Could you check a few things on this model? Use its own coordinates, in mm. Face numbers are marked on the shaded views. A direction names the side the tool comes from. Round coordinates to 2 decimals unless told otherwise and drop trailing zeros. Loops run counter-clockwise (first coordinate to the right, second up) from the corner with the lowest first, then second, coordinate; pieces in that order, holes last. Notation, with made-up numbers: (-19.75, 75) -> (39.25, 75) arc R4 ccw to (39.25, 82) -> close; hole circle Ø3 at (11, 81). An arc over 180 degrees is marked (long way). One line per item, written item: value.
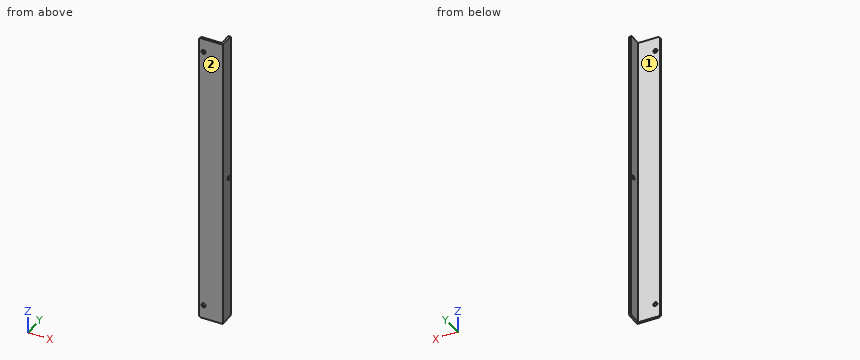
```python
from build123d import *

# Parameters (mm, degrees)
BOSS_EXTRUDE1_DEPTH = 750
CUT_EXTRUDE1_REACH  = 755.21
SKETCH4_R           = 5.25
CUT_EXTRUDE2_REACH  = 755.077
SKETCH5_R           = 5.25
CHAMFER1_SIZE       = 4


with BuildPart() as part:
    # Sketch1 → Boss-Extrude1 (new body)
    with BuildSketch(Plane.XY):
        Polygon((0, 0), (-60, 0), (-60, 5), (-5, 5), (-5, 40), (0, 40), align=None)
    extrude(amount=BOSS_EXTRUDE1_DEPTH)

    # Sketch4 → Cut-Extrude1 (cut, up to next)
    with BuildSketch(Plane(origin=(0, 5, 0), x_dir=(1, 0, 0), z_dir=(0, 1, 0)), mode=Mode.PRIVATE) as cut_extrude1_sk1:
        with Locations(Location((-48, -35, 0), (0, 0, 270))):
            Circle(SKETCH4_R)
    cut_extrude1_tool1 = extrude(cut_extrude1_sk1.sketch, amount=-CUT_EXTRUDE1_REACH, mode=Mode.PRIVATE) & part.part
    # Sketch4 → Cut-Extrude1 (cut, up to next)
    with BuildSketch(Plane(origin=(0, 5, 0), x_dir=(1, 0, 0), z_dir=(0, 1, 0)), mode=Mode.PRIVATE) as cut_extrude1_sk2:
        with Locations(Location((-48, -715, 0), (0, 0, 180))):
            Circle(SKETCH4_R)
    cut_extrude1_tool2 = extrude(cut_extrude1_sk2.sketch, amount=-CUT_EXTRUDE1_REACH, mode=Mode.PRIVATE) & part.part
    add(cut_extrude1_tool1.solids().sort_by_distance((-48, 5, 35))[0], mode=Mode.SUBTRACT)
    add(cut_extrude1_tool2.solids().sort_by_distance((-48, 5, 715))[0], mode=Mode.SUBTRACT)

    # Sketch5 → Cut-Extrude2 (cut, up to next)
    with BuildSketch(Plane.ZY.offset(5), mode=Mode.PRIVATE) as cut_extrude2_sk1:
        with Locations(Location((375, 28, 0), (0, 0, 270))):
            Circle(SKETCH5_R)
    cut_extrude2_tool1 = extrude(cut_extrude2_sk1.sketch, amount=-CUT_EXTRUDE2_REACH, mode=Mode.PRIVATE) & part.part
    add(cut_extrude2_tool1.solids().sort_by_distance((-5, 28, 375))[0], mode=Mode.SUBTRACT)

    # Chamfer1
    chamfer1_edges = [part.edges().sort_by_distance(p)[0] for p in [
        (-60, 2.5, 750),
        (-60, 2.5, 0),
        (-2.5, 40, 750),
        (-2.5, 40, 0),
    ]]
    chamfer(chamfer1_edges, length=CHAMFER1_SIZE)


solid = part.part
```
Item 1: I need wall thicknesses on line 1 (Z direction, x = -4, y = 29); line 2 (X direction, y = 3.9, z = 35); line 3 (Y direction, x = -40, z = 504). Which ranges of each line are inside material? Lowest first, please. Write a range as from..to.
Output:
line 1: z = 0..369.85, 380.15..750
line 2: x = -60..-53.25, -42.75..0
line 3: y = 0..5
Item 2: If we section it at C-C on x = -24: List the corners of the cut face in (y, z) for me, plus the area to 3 significant figures.
Output:
outline: (0, 0) -> (5, 0) -> (5, 750) -> (0, 750) -> close
area: 3,750 mm²
Item 3: If we section it at B-B on y = 14.5: List the corners of the cut face in (x, z) for me.
Output:
outline: (-5, 0) -> (0, 0) -> (0, 750) -> (-5, 750) -> close
Item 4: Will these pins go through, and if not, where does the flat tip stop? pin 1 Ø6.5 at (x, z) = (-48, 35) entering from -Y; pin 2 Ø6 at (x, z) = (-38.5, 371.5) entering from +Y.
Output:
pin 1: passes through
pin 2: stops at y = 5
Item 5: If we section it at A-A on z = 258: List the corners of the cut face in (x, y) for me, plus the area to 3 significant figures.
Output:
outline: (-60, 0) -> (0, 0) -> (0, 40) -> (-5, 40) -> (-5, 5) -> (-60, 5) -> close
area: 475 mm²
Item 6: For the marked faces 1 and 2, which set-ups out of +Z, -Z, +X, -X, +Y, -Y let a thin tool reach every point of the face, with its end or its side?
Output:
face 1: +Z, -Z, -X, +Y
face 2: +Z, -Z, +X, -X, -Y
